```python
from build123d import *

# Parameters (mm, degrees)
SKETCH_1_W          = 52
SKETCH_1_H          = 54
EXTRUDE_1_DEPTH     = 47
CUT_EXTRUDE_START   = 47
SKETCH_2_W          = 40
SKETCH_2_H          = 46
CUT_EXTRUDE_1_DEPTH = 43
CUT_EXTRUDE_START_2 = -20
SKETCH_4_R          = 11.2
SKETCH_4_R_2        = 1.75
CUT_EXTRUDE_3_DEPTH = 6
SKETCH_5_W          = 40
SKETCH_5_H          = 14
SKETCH_5_R          = 3
EXTRUDE_2_DEPTH     = 6
FILLET_1_R          = 6


with BuildPart() as part:
    # 草图1 → 凸台-拉伸1 (new body)
    with BuildSketch(Plane(origin=(0, 0, 0), x_dir=(1, 0, 0), z_dir=(0, 1, 0))):
        Rectangle(SKETCH_1_W, SKETCH_1_H)
    extrude(amount=EXTRUDE_1_DEPTH)

    # 草图2 → 切除-拉伸1 (cut)
    with BuildSketch(Plane(origin=(0, 0, 0), x_dir=(1, 0, 0), z_dir=(0, 1, 0)).offset(CUT_EXTRUDE_START)):
        Rectangle(SKETCH_2_W, SKETCH_2_H)
    extrude(amount=-CUT_EXTRUDE_1_DEPTH, mode=Mode.SUBTRACT)

    # 草图4 → 切除-拉伸3 (cut)
    with BuildSketch(Plane(origin=(0, 0, 0), x_dir=(0, 0, -1), z_dir=(1, 0, 0)).offset(CUT_EXTRUDE_START_2)):
        with Locations((0, 25)):
            Circle(SKETCH_4_R)
        with Locations((-15.5, 40.5)):
            Circle(SKETCH_4_R_2)
        with Locations((15.5, 40.5)):
            Circle(SKETCH_4_R_2)
        with Locations((15.5, 9.5)):
            Circle(SKETCH_4_R_2)
        with Locations((-15.5, 9.5)):
            Circle(SKETCH_4_R_2)
    extrude(amount=-CUT_EXTRUDE_3_DEPTH, mode=Mode.SUBTRACT)

    # 草图5 → 凸台-拉伸2 (add)
    # profile 1 of 2: a face of its own
    with BuildSketch(Plane(origin=(0, 0, 0), x_dir=(1, 0, 0), z_dir=(0, 1, 0))):
        with Locations((0, 34)):
            Rectangle(SKETCH_5_W, SKETCH_5_H)
        with Locations(Location((-10, 34, 0), (0, 0, 270))):
            Circle(SKETCH_5_R, mode=Mode.SUBTRACT)
        with Locations(Location((10, 34, 0), (0, 0, 270))):
            Circle(SKETCH_5_R, mode=Mode.SUBTRACT)
    # profile 2 of 2: a face of its own
    with BuildSketch(Plane(origin=(0, 0, 0), x_dir=(1, 0, 0), z_dir=(0, 1, 0))):
        with Locations((0, -34)):
            Rectangle(SKETCH_5_W, SKETCH_5_H)
        with Locations(Location((10, -34, 0), (0, 0, 90))):
            Circle(SKETCH_5_R, mode=Mode.SUBTRACT)
        with Locations(Location((-10, -34, 0), (0, 0, 90))):
            Circle(SKETCH_5_R, mode=Mode.SUBTRACT)
    extrude(amount=EXTRUDE_2_DEPTH)

    # 圆角1
    fillet_1_edges = [part.edges().sort_by_distance(p)[0] for p in [
        (-20, 3, -41),
        (20, 3, -41),
        (-20, 3, 41),
        (20, 3, 41),
    ]]
    fillet(fillet_1_edges, radius=FILLET_1_R)


solid = part.part
```
Here's how the part is built. I have some questions about the finished solid (model axes, mm). A direction names the side the tool comes from. Give positions to 0.01 mm unless a question says otherwise; leave off trailing zeros. Loops run counter-clockwise (first coordinate to the right, second up) from the corner with the lowest first, then second, coordinate; pieces in that order, holes last. Notation, with made-up numbers: (1.25, 89.5) -> (12.25, 89.5) arc R15 ccw to (12.25, 98.5) -> close; hole circle Ø9 at (8, 33). An arc over 180 degrees is marked (long way). Use one line per item in the form item = value. Start each with the question number.
1) Which directions (+Z, -Z, +X, -X, +Y, -Y) give clear straight access to the entire face, cutting with the end or side of a thin tool? Please do faces 1 (the face through (-20, 35.4, 5.4)), 2 (the face through (0, 3, 41)), 3 (the face through (0, 6, -34)), 4 (the face through (-22.96, 38.95, 14.69)), 5 (the face through (-20, 3, 31)).
2) For P1, Ø7, axis at x = 5, z = -32, coming from the +Y side; P2, Ø1.8, axis at y = 2.5, z = 32, coming from the -X side; P3, Ø6, axis at x = 2.5, z = -6, coming from the +Y side; P4, Ø5, axis at x = -10, z = -34, coming from the +Y side, each with a flat end and sliding along its axis, tell me the tip position at first contact or that it passes through.
3) Please list where these lines run through material, in increasing order: line 1 along Y through (x, z) = (-22.2, -15.5); line 2 along X through (y, z) = (43.5, -12); line 3 along X through (y, z) = (1.5, -34).
4) Imagine slicing it at C-C (x = 3.5). Please give me the cut outline in (y, z), then the cut area to 3 significant figures.
5) Imagine slicing it at B-B (x = 10). Please give me the cut outline in (y, z), then the cut area to 3 significant figures.
6) Imagine slicing it at D-D (z = 34). Please give me the cut outline in (x, y), then the cut area to 3 significant figures.
7) Thinking about a two-plate mould opening in X: for faces 6 (the face through (0, 3, -41)), 7 (the face through (10, 3, -37)), 8 (the face through (0, 26, 23)), 9 (the face through (-20, 3, -31)), which applies, +X half, -X half, draft (parallel to the pull), parting line (faces both ways), or undercut?
8) Imagine slicing it at A-A (z = -15.5). Please give me the cut outline in (x, y).
Check values:
q1.face_1 = +Y
q1.face_2 = +Z, +X, -X, +Y, -Y
q1.face_3 = -Z, +X, -X, +Y
q1.face_4 = -X
q1.face_5 = +Z, -X, +Y, -Y
q2.P1 = 6
q2.P2 = -20
q2.P3 = 4
q2.P4 = through
q3.line_1 = 0 to 7.75, 11.25 to 38.75, 42.25 to 47
q3.line_2 = -26 to -20, 20 to 26
q3.line_3 = -20 to -13, -7 to 7, 13 to 20
q4.outline = (0, -41) -> (6, -41) -> (6, -27) -> (47, -27) -> (47, -23) -> (4, -23) -> (4, 23) -> (47, 23) -> (47, 27) -> (6, 27) -> (6, 41) -> (0, 41) -> close
q4.area = 728 mm^2
q5.outline = (0, -41) -> (6, -41) -> (6, -37) -> (0, -37) -> close; (0, -31) -> (6, -31) -> (6, -27) -> (47, -27) -> (47, -23) -> (4, -23) -> (4, 23) -> (47, 23) -> (47, 27) -> (6, 27) -> (6, 31) -> (0, 31) -> close; (0, 37) -> (6, 37) -> (6, 41) -> (0, 41) -> close
q5.area = 656 mm^2
q6.outline = (-20, 0) -> (-13, 0) -> (-13, 6) -> (-20, 6) -> close; (-7, 0) -> (7, 0) -> (7, 6) -> (-7, 6) -> close; (13, 0) -> (20, 0) -> (20, 6) -> (13, 6) -> close
q6.area = 168 mm^2
q7.face_6 = draft
q7.face_7 = undercut
q7.face_8 = undercut
q7.face_9 = -X half
q8.outline = (-26, 0) -> (26, 0) -> (26, 47) -> (20, 47) -> (20, 4) -> (-20, 4) -> (-20, 7.75) -> (-26, 7.75) -> close; (-26, 11.25) -> (-20, 11.25) -> (-20, 38.75) -> (-26, 38.75) -> close; (-26, 42.25) -> (-20, 42.25) -> (-20, 47) -> (-26, 47) -> close
